from build123d import *

# Parameters (mm, degrees)
F1_DEPTH      = 19.05
F3_D          = 6.35
F4_W          = 1.5875
F4_H          = 35.8877405588
F5_DEPTH      = 25.4
F5_DEPTH_BACK = 1.27
F6_R          = 15.875
F7_DEPTH      = 3.81
F8_W          = 11.7475
F8_H          = 3.175
F9_DEPTH      = 25.4
F10_W         = 11.7475
F10_H         = 3.175
F11_DEPTH     = 25.4


with BuildPart() as f1:
    # F0 (on Right) → F1 (new body)
    with BuildSketch(Plane.YZ):
        with BuildLine():
            ThreePointArc((-3.9967504682, -1.0709260603), (-1.8851834207, 0.7808685404), (-2.0688702794, 3.5833884382))
            Line((-2.0688702794, 3.5833884382), (-36.2669128953, 62.8161357684))
            ThreePointArc((-36.2669128953, 62.8161357684), (-38.5911742094, 65.1403970824), (-41.7661742094, 65.9911357684))
            Line((-41.7661742094, 65.9911357684), (-47.625, 65.9911357684))
            Line((-47.625, 65.9911357684), (-47.625, 59.6411357684))
            Line((-47.625, 59.6411357684), (-44.45, 59.6411357684))
            ThreePointArc((-44.45, 59.6411357684), (-39.9598719395, 57.7812638289), (-38.1, 53.2911357684))
            Line((-38.1, 53.2911357684), (-38.1, 2.4911357684))
            ThreePointArc((-38.1, 2.4911357684), (-39.9598719395, -1.9989922922), (-44.45, -3.8588642316))
            Line((-44.45, -3.8588642316), (-47.625, -3.8588642316))
            Line((-47.625, -3.8588642316), (-47.625, -10.2088642316))
            Line((-47.625, -10.2088642316), (-38.9359933597, -10.2088642316))
            ThreePointArc((-38.9359933597, -10.2088642316), (-38.1071520391, -10.1545391013), (-37.2924924233, -9.9924932286))
            Line((-37.2924924233, -9.9924932286), (-3.9967504682, -1.0709260603))
        make_face()
    extrude(amount=F1_DEPTH)

    # F3 (through all)
    with Locations(Plane(origin=(0, 0, -10.2088642316), x_dir=(1, 0, 0), z_dir=(0, 0, -1))):
        with Locations((9.525, 42.8625)):
            Hole(F3_D / 2)

    # F4 (on Top) → F5 (cut, two sides)
    with BuildSketch(Plane.XY) as f5_sk:
        with Locations((9.525, 0)):
            Rectangle(F4_W, F4_H)
    extrude(amount=-F5_DEPTH, mode=Mode.SUBTRACT)
    extrude(f5_sk.sketch, amount=F5_DEPTH_BACK, mode=Mode.SUBTRACT)

    # F6 (on Top) → F7 (cut)
    with BuildSketch(Plane.XY):
        with Locations((9.525, -1.5875)):
            Circle(F6_R)
    extrude(amount=F7_DEPTH, mode=Mode.SUBTRACT)

    # F8 (on face) → F9 (cut)
    with BuildSketch(Plane.XZ.offset(47.625)):
        with Locations((9.525, 65.9911357684)):
            Rectangle(F8_W, F8_H)
    extrude(amount=-F9_DEPTH, mode=Mode.SUBTRACT)

    # F10 (on face) → F11 (cut)
    with BuildSketch(Plane.XZ.offset(47.625)):
        with Locations((9.525, -10.2088642316)):
            Rectangle(F10_W, F10_H)
    extrude(amount=-F11_DEPTH, mode=Mode.SUBTRACT)


solid = f1.part
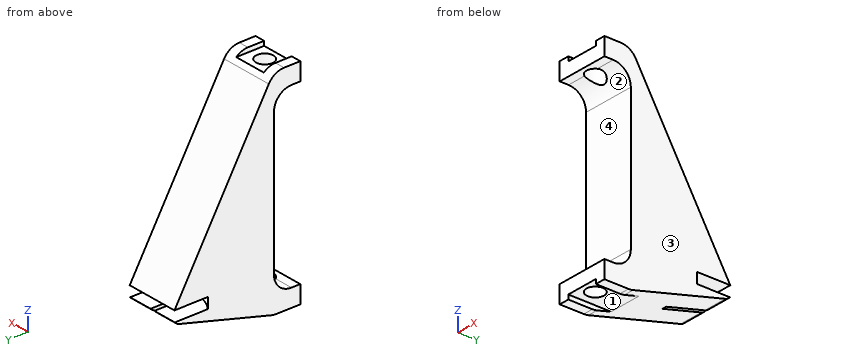
The listing builds one solid part. Answer for the finished solid, in the listing's coordinates (mm). Face numbers are marked on the shaded views. Coordinates: 2 decimals unless noted, no trailing zeros. Order: outer loops, then holes, each group sorted by start corner. A loop starts at its lowest first (then second) coordinate and runs counter-clockwise, first axis right, second up.
Q1. A cutting plane is placed at B-B, the plane x = 11.5. State how many separate pieces and enclosed holes the cut face has, and give its area (3 significant figures).
Q2. For a pull along Z with two mould halves and no side action, classify the marked faces 1, 2, 3 and 4 as pulls with the +Z half, pulls with the -Z half, needs draft (parallel to the pull), parting line crosses it, or undercut.
Q3. Consider line 1 (Z direction, x = 2.25, y = -12); line 2 (Z direction, x = 16.75, y = -5.5); line 3 (Z direction, x = 16.5, y = -24.5). Determine where each line is inside the solid, lowest interval first.
Q4. A cutting plane is placed at A-A, the plane y = -7. Write down the section's boundary in (x, z).
Q5. A cutting plane is placed at C-C, the plane y = -35. Write down the section's boundary in (x, z), and give its area (3 significant figures).
Q6. Given P1, Ø9.5, axis at x = 4.5, y = -8, coming from the +Z side; P2, Ø10, axis at x = 11, z = 40.5, coming from the +Y side; P3, Ø2.5, axis at x = 6.5, y = -46.5, coming from the +Z side; P4, Ø0.5, axis at y = -43.5, z = -9.5, coming from the -X side, each flat-ended and moving along its own axis, determine where each tip first touches the part or whether it passes through.
Answers follow:
1. separate pieces: 3
1. enclosed holes: 0
1. area: 1,440 mm2
2. face 1: pulls with the -Z half
2. face 2: undercut
2. face 3: needs draft
2. face 4: undercut
3. line 1: z = -3.22 to 0, 3.81 to 20.78
3. line 2: z = -1.47 to 0, 3.81 to 9.53
3. line 3: z = -6.56 to 42.44
4. outline: (0, -1.88) - (8.73, -1.88) - (8.73, 0) - (0, 0) - close; (0, 3.81) - (19.05, 3.81) - (19.05, 12.12) - (0, 12.12) - close; (10.32, -1.88) - (19.05, -1.88) - (19.05, 0) - (10.32, 0) - close
5. outline: (0, -9.38) - (3.65, -9.38) - (3.65, -8.62) - (15.4, -8.62) - (15.4, -9.38) - (19.05, -9.38) - (19.05, 60.62) - (0, 60.62) - close
5. area: 1,320 mm2
6. P1: stops at z = 22.08
6. P2: stops at y = -20.5
6. P3: stops at z = 64.4
6. P4: stops at x = 0
